Verification items for the finished model (mm, model axes). A direction names the side the tool comes from. Coordinates: 2 decimals unless noted, no trailing zeros. Write each loop counter-clockwise with the first axis right and the second up, starting at its lowest first coordinate (ties: lowest second). Pieces come first, ordered by that corner, then holes. Notation, with made-up numbers: (78.5, -39.5) -> (87.5, -39.5) arc R14 ccw to (87.5, -18.5) -> close; hole circle Ø7 at (-19, 86.5). An arc over 180 degrees is marked (long way). Write each question's results on one line, items separated by ' | '. Start each with the question number.
from build123d import *

# Parameters (mm, degrees)
F0_W     = 914.4
F0_H     = 2133.6
F1_DEPTH = 152.4
F2_R     = 12.7
F3_R     = 5.08


# Not quite as in the source:
# - a feature names something its author has since deleted; it is built from what else it names


with BuildPart() as f1:
    # F0 (on Front) → F1 (new body)
    with BuildSketch(Plane.XZ):
        with Locations((457.2, 1066.8)):
            Rectangle(F0_W, F0_H)
        Polygon((330.2, 1737.36), (457.2, 1737.36), (584.2, 1737.36), (584.2, 1483.36), (330.2, 1483.36), align=None, mode=Mode.SUBTRACT)
    extrude(amount=F1_DEPTH)

    # F2
    f2_edges = [f1.edges().sort_by_distance(p)[0] for p in [
        (457.2, -152.4, 2133.6),
        (914.4, -152.4, 1066.8),
        (914.4, -76.2, 2133.6),
        (457.2, 0, 2133.6),
        (914.4, 0, 1066.8),
        (914.4, -76.2, 0),
        (457.2, -152.4, 0),
        (0, -152.4, 1066.8),
        (457.2, 0, 0),
        (0, 0, 1066.8),
        (0, -76.2, 0),
        (0, -76.2, 2133.6),
    ]]
    fillet(f2_edges, radius=F2_R)

    # F3
    f3_edges = [f1.edges().sort_by_distance(p)[0] for p in [
        (457.2, -152.4, 1483.36),
        (330.2, -152.4, 1610.36),
        (457.2, -152.4, 1737.36),
        (457.2, 0, 1483.36),
        (330.2, 0, 1610.36),
        (584.2, 0, 1610.36),
        (457.2, 0, 1737.36),
        (584.2, -152.4, 1610.36),
        (584.2, -76.2, 1483.36),
        (330.2, -76.2, 1483.36),
        (330.2, -76.2, 1737.36),
        (584.2, -76.2, 1737.36),
    ]]
    fillet(f3_edges, radius=F3_R)


solid = f1.part
1. Mould release check, pull along Z, two halves, no side actions. Record for faces 3 (the flat face through (451, -152.4, 1082)), 4 (the flat face through (451, -75, 2133.6)), 5 (the flat face through (584.2, -75, 1612)), 6 (the flat face through (330.2, -75, 1609)): +Z half, -Z half, draft (parallel to the pull), parting line (faces both ways), or undercut.
2. Tool access check on faces 1 (the flat face through (451, -75, 0)), 2 (the flat face through (459, -75, 1483.36)). Record the directions out of +Z, -Z, +X, -X, +Y, -Y that give a thin tool (end or side, any length) a straight path to the whole face; none if there is none.
3. Sectioned sample at A-A on x = 503.5. Record the cut outline in (y, z), plus the area to 3 significant figures.
4. Sectioned sample at B-B on y = -70. Record the cut outline in (x, z).
5. Material ranges on probe 1 along Z at (x, y) = (430, -68.5); probe 2 along Z at (x, y) = (581, -77); probe 3 along X at (y, z) = (-144, 1729), recorded low to high. Write a range as from..to.
Computed values:
1) face 3: draft | face 4: +Z half | face 5: undercut | face 6: undercut
2) face 1: -Z, +X, -X, +Y, -Y | face 2: +Y, -Y
3) outline: (-152.4, 12.7) arc R12.7 ccw to (-139.7, 0) -> (-12.7, 0) arc R12.7 ccw to (0, 12.7) -> (0, 1478.28) arc R5.08 ccw to (-5.08, 1483.36) -> (-147.32, 1483.36) arc R5.08 ccw to (-152.4, 1478.28) -> close; (-152.4, 1742.44) arc R5.08 ccw to (-147.32, 1737.36) -> (-5.08, 1737.36) arc R5.08 ccw to (0, 1742.44) -> (0, 2120.9) arc R12.7 ccw to (-12.7, 2133.6) -> (-139.7, 2133.6) arc R12.7 ccw to (-152.4, 2120.9) -> close | area: 286,000 mm^2
4) outline: (0, 12.7) arc R12.7 ccw to (12.7, 0) -> (901.7, 0) arc R12.7 ccw to (914.4, 12.7) -> (914.4, 2120.9) arc R12.7 ccw to (901.7, 2133.6) -> (12.7, 2133.6) arc R12.7 ccw to (0, 2120.9) -> close; hole (330.2, 1488.44) arc R5.08 ccw to (335.28, 1483.36) -> (579.12, 1483.36) arc R5.08 ccw to (584.2, 1488.44) -> (584.2, 1732.28) arc R5.08 ccw to (579.12, 1737.36) -> (335.28, 1737.36) arc R5.08 ccw to (330.2, 1732.28) -> close
5) probe 1: z = 0..1483.36, 1737.36..2133.6 | probe 2: z = 0..1483.72, 1737..2133.6 | probe 3: x = 0.75..330.2, 584.2..913.65
